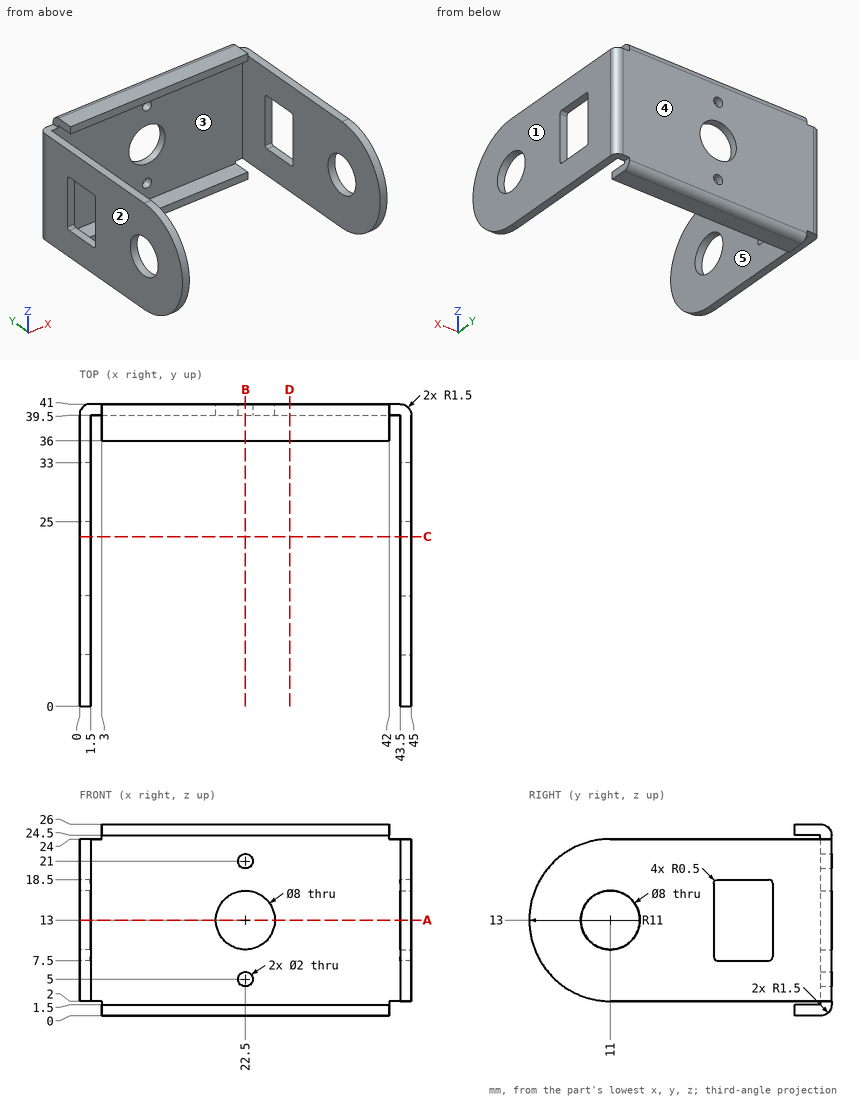
Check sheet for the drawn part. Datum: minimum x, y, z corner. Units: mm. A direction names the side the tool comes from. Round coordinates to 2 decimals unless told otherwise and drop trailing zeros. Order: outer loops, then holes, each group sorted by start corner. A loop starts at its lowest first (then second) coordinate and runs counter-clockwise, first axis right, second up.
1) Mould release check, pull along X, two halves, no side actions. Record for the marked faces 1, 2 and 3: +X half, -X half, draft (parallel to the pull), parting line (faces both ways), or undercut.
2) Section check D-D (x = 28.5). Record the boundary of the cut face in (y, z), and give its area (3 significant figures).
3) Scan lines: line 1 (X direction, y = 24.5, z = 17.25); line 2 (Z direction, x = 22.5, y = 40.05); line 3 (Z direction, x = 22.5, y = 40.45). Record each from-to range of solid material in increasing order.
4) Section check A-A (z = 13). Give the number of separate pieces and of enclosed holes in the cut face, and give its area (3 significant figures).
5) Tool access check on the marked faces 4 and 5. Record the directions out of +Z, -Z, +X, -X, +Y, -Y that give a thin tool (end or side, any length) a straight path to the whole face; none if there is none.
6) Section check B-B (x = 22.5). Record the boundary of the cut face in (y, z).
7) Section check C-C (y = 23). Record the boundary of the cut face in (x, z), and give its area (3 significant figures).
8) Go/stop test with flat-tipped pins: pin 1 Ø8 at (x, y) = (8, 26) entering from -Z; pin 2 Ø3.5 at (x, y) = (1.5, 20) entering from -Z; pin 3 Ø1.6 at (y, z) = (38, 25) entering from +X; pin 4 Ø0.9 at (x, y) = (43.5, 21.5) entering from +Z. Record where each tip stops, or that it passes through.
Result:
1. face 1: +X half
1. face 2: -X half
1. face 3: undercut
2. outline: (36, 0) - (39.5, 0) arc R1.5 ccw to (41, 1.5) - (41, 24.5) arc R1.5 ccw to (39.5, 26) - (36, 26) - (36, 24.5) - (39.5, 24.5) - (39.5, 1.5) - (36, 1.5) - close
2. area: 48.5 mm2
3. line 1: x = 0 to 1.5, 43.5 to 45
3. line 2: z = 0.1 to 4, 6 to 9, 17 to 20, 22 to 25.9
3. line 3: z = 0.34 to 4, 6 to 9, 17 to 20, 22 to 25.66
4. separate pieces: 6
4. enclosed holes: 0
4. area: 125 mm2
5. face 4: +Z, -Z, +X, -X, +Y
5. face 5: +Z, -Z, -Y
6. outline: (36, 0) - (39.5, 0) arc R1.5 ccw to (41, 1.5) - (41, 4) - (39.5, 4) - (39.5, 1.5) - (36, 1.5) - close; (36, 24.5) - (39.5, 24.5) - (39.5, 22) - (41, 22) - (41, 24.5) arc R1.5 ccw to (39.5, 26) - (36, 26) - close; (39.5, 6) - (41, 6) - (41, 9) - (39.5, 9) - close; (39.5, 17) - (41, 17) - (41, 20) - (39.5, 20) - close
7. outline: (0, 2) - (1.5, 2) - (1.5, 24) - (0, 24) - close; (43.5, 2) - (45, 2) - (45, 24) - (43.5, 24) - close
7. area: 66.0 mm2
8. pin 1: passes through
8. pin 2: stops at z = 2
8. pin 3: stops at x = 42
8. pin 4: stops at z = 24
